Could you check a few things on this model? Use its own coordinates, in mm. A direction names the side the tool comes from. Give positions to 0.01 mm unless a question says otherwise; leave off trailing zeros. Loops run counter-clockwise (first coordinate to the right, second up) from the corner with the lowest first, then second, coordinate; pieces in that order, holes last. Notation, with made-up numbers: (84, 5) - (124, 5) arc R30 cw to (124, 31) - close; hole circle Ø5 at (60, 87.5). An arc over 180 degrees is marked (long way). Answer in a Markdown table with one row per item. Add a question column.
```python
from build123d import *

# Parameters (mm, degrees)
SKETCH1_W           = 70.5
SKETCH1_H           = 70.5
SKETCH1_W_2         = 60.5
SKETCH1_H_2         = 60.5
BOSS_EXTRUDE1_DEPTH = 10
SKETCH2_W           = 67
SKETCH2_H           = 5.4
CUT_EXTRUDE1_DEPTH  = 70
BOSS_EXTRUDE3_DEPTH = 2
SKETCH7_W           = 60.5
SKETCH7_H           = 5
CUT_EXTRUDE3_DEPTH  = 25
FILLET2_R           = 2
SKETCH8_W           = 97.382964501
SKETCH8_H           = 35.083557697
CUT_EXTRUDE4_DEPTH  = 2
SKETCH9_R           = 2.15
CUT_EXTRUDE5_DEPTH  = 5
SKETCH10_R          = 3.5
CUT_EXTRUDE6_DEPTH  = 8
FILLET3_R           = 10
FILLET4_R           = 10
FILLET5_R           = 1


# Some blends are built 0.0001 mm under size
with BuildPart() as part:
    # Sketch1 → Boss-Extrude1 (new body)
    with BuildSketch(Plane(origin=(0, 0, 0), x_dir=(1, 0, 0), z_dir=(0, 1, 0))):
        Rectangle(SKETCH1_W, SKETCH1_H)
        Rectangle(SKETCH1_W_2, SKETCH1_H_2, mode=Mode.SUBTRACT)
    extrude(amount=BOSS_EXTRUDE1_DEPTH)

    # Sketch2 → Cut-Extrude1 (cut)
    with BuildSketch(Plane.XY.offset(35.25)):
        Rectangle(SKETCH2_W, SKETCH2_H)
    extrude(amount=-CUT_EXTRUDE1_DEPTH, mode=Mode.SUBTRACT)

    # Sketch6 → Boss-Extrude3 (add)
    with BuildSketch(Plane.XZ):
        Polygon((41.25, -37.25), (41.25, 37.25), (35.25, 37.25), (35.25, 35.25), (35.25, -35.25), (-35.25, -35.25), (-35.25, 35.25), (-35.25, 37.25), (-41.25, 37.25), (-41.25, -37.25), align=None)
    extrude(amount=-BOSS_EXTRUDE3_DEPTH)

    # Sketch7 → Cut-Extrude3 (cut)
    with BuildSketch(Plane.XZ.offset(-2.7)):
        with Locations((0, 32.75)):
            Rectangle(SKETCH7_W, SKETCH7_H)
    extrude(amount=-CUT_EXTRUDE3_DEPTH, mode=Mode.SUBTRACT)

    # Fillet2
    fillet2_edges = [part.edges().sort_by_distance(p)[0] for p in [
        (35.25, 2, 0),
        (-35.25, 2, 0),
        (0, 2, -35.25),
    ]]
    fillet(fillet2_edges, radius=FILLET2_R - 0.0001)  # a hair under: the kernel refuses the full size

    # Sketch8 → Cut-Extrude4 (cut)
    with BuildSketch(Plane.XY.offset(37.25)):
        with Locations((-5.820498703, 2.430952297)):
            Rectangle(SKETCH8_W, SKETCH8_H)
    extrude(amount=-CUT_EXTRUDE4_DEPTH, mode=Mode.SUBTRACT)

    # Sketch9 → Cut-Extrude5 (cut, symmetric)
    with BuildSketch(Plane.XZ):
        with Locations(Location((-37.375, 25.25, 0), (0, 0, 273.333029494))):
            Circle(SKETCH9_R)
        with Locations(Location((-37.375, -19.75, 0), (0, 0, 273.333029494))):
            Circle(SKETCH9_R)
        with Locations(Location((37.375, -19.75, 0), (0, 0, 266.666970506))):
            Circle(SKETCH9_R)
        with Locations(Location((37.375, 25.25, 0), (0, 0, 266.666970506))):
            Circle(SKETCH9_R)
    extrude(amount=CUT_EXTRUDE5_DEPTH, both=True, mode=Mode.SUBTRACT)

    # Sketch10 → Cut-Extrude6 (cut)
    with BuildSketch(Plane(origin=(0, 10, 0), x_dir=(1, 0, 0), z_dir=(0, 1, 0))):
        with Locations((-37.375, 19.75)):
            Circle(SKETCH10_R)
        with Locations((-37.375, -25.25)):
            Circle(SKETCH10_R)
        with Locations((37.375, -25.25)):
            Circle(SKETCH10_R)
        with Locations((37.375, 19.75)):
            Circle(SKETCH10_R)
    extrude(amount=-CUT_EXTRUDE6_DEPTH, mode=Mode.SUBTRACT)

    # Fillet3
    # the kernel refuses this fillet: 10 mm, written as the material it takes off along each edge
    with BuildSketch(Plane(origin=(-33.5, -24.358969087, 35.25), x_dir=(0, 0, -1), z_dir=(0, 1, 0)), Plane(origin=(33.5, 2.7, 35.25), x_dir=(0, 0, -1), z_dir=(0, -1, 0))) as fillet3_piece_1:
        with BuildLine():
            CenterArc((9.743587635, 10), FILLET3_R, 193.002878163, 76.997121837)
            Line((0, 7.75), (0, 0))
            Line((0, 0), (9.743587635, 0))
        make_face()
    extrude(amount=27.058969087, mode=Mode.SUBTRACT)

    # Fillet4
    # the kernel refuses this fillet: 10 mm, written as the material it takes off along each edge
    with BuildSketch(Plane(origin=(30.25, -18.950635095, 35.25), x_dir=(0, 0, -1), z_dir=(0, 1, 0))) as fillet4_piece_1:
        with BuildLine():
            CenterArc((8.660254038, -10), FILLET4_R, 90, 60)
            Line((0, -5), (-0.173205081, -4.9))
            ThreePointArc((-0.173205081, -4.9), (-0.2, -2.5), (-0.2, 0))
            Line((-0.2, 0), (0, 0.2))
            Line((0, 0.2), (8.660254038, 0.2))
            Line((8.660254038, 0.2), (8.660254038, 0))
        make_face()
    extrude(amount=50.601270189, mode=Mode.SUBTRACT)
    with BuildSketch(Plane(origin=(-30.25, -18.950635095, 35.25), x_dir=(0, 0, -1), z_dir=(0, 1, 0))) as fillet4_piece_2:
        with BuildLine():
            CenterArc((8.660254038, 10), FILLET4_R, 210, 60)
            Line((0, 5), (-0.173205081, 4.9))
            ThreePointArc((-0.173205081, 4.9), (-0.2, 2.5), (-0.2, 0))
            Line((-0.2, 0), (0, -0.2))
            Line((0, -0.2), (8.660254038, -0.2))
            Line((8.660254038, -0.2), (8.660254038, 0))
        make_face()
    extrude(amount=50.601270189, mode=Mode.SUBTRACT)

    # Fillet5
    # the kernel refuses this fillet: 1 mm, written as the material it takes off along each edge
    with BuildSketch(Plane(origin=(30.25, 2.7, 26.589745962), x_dir=(1, 0, 0), z_dir=(0, 0, -1)), Plane(origin=(-30.25, 2.7, -30.25), x_dir=(-1, 0, 0), z_dir=(0, 0, 1))) as fillet5_piece_1:
        with BuildLine():
            CenterArc((FILLET5_R, -FILLET5_R), FILLET5_R, 90, 90)
            Line((0, -FILLET5_R), (0, 0))
            Line((0, 0), (FILLET5_R, 0))
        make_face()
    extrude(amount=56.839745962, mode=Mode.SUBTRACT)
    with BuildSketch(Plane(origin=(40.25, 2.7, 26.589745962), x_dir=(-0.27015512952929444, 0, 0.9628168081151316), z_dir=(0.9628168081151316, 0, 0.27015512952929444))) as fillet5_piece_2:
        with BuildLine():
            CenterArc((10 - FILLET5_R, -FILLET5_R), FILLET5_R, 0, 90)
            Line((10 - FILLET5_R, 0), (10, 0))
            Line((10, 0), (10, -FILLET5_R))
        make_face()
    revolve(axis=Axis((40.25, 2.7, 26.589745962), (0, -1, 0)), revolution_arc=74.326501832, mode=Mode.SUBTRACT)
    with BuildSketch(Plane(origin=(-40.25, 2.7, 26.589745962), x_dir=(1, 0, 0), z_dir=(0, 0, -1))) as fillet5_piece_3:
        with BuildLine():
            CenterArc((10 - FILLET5_R, -FILLET5_R), FILLET5_R, 0, 90)
            Line((10, -FILLET5_R), (10, 0))
            Line((10, 0), (10 - FILLET5_R, 0))
        make_face()
    revolve(axis=Axis((-40.25, 2.7, 26.589745962), (0, -1, 0)), revolution_arc=74.326501832, mode=Mode.SUBTRACT)


solid = part.part
```
(1) I want a section at D-D on y = 5.75. Please give me the cut outline in (x, z) (3 decimals), then the cut area to 3 significant figures.
(2) For pin 1 Ø3 at (y, z) = (7.5, -31) entering from -X; pin 2 Ø6 at (x, y) = (-16, 5) entering from +Z; pin 3 Ø1 at (y, z) = (3, 12) entering from -X; pin 4 Ø3.5 at (x, z) = (-37.375, 25.25) entering from +Y, each with a flat end and sliding along its axis, tell me the tip position at first contact or that it passes through.
(3) Please list where these lines run through material, in increasing order: line 1 (X direction, y = 0.9, z = -19.75) (3 decimals); line 2 (X direction, y = 7, z = -5); line 3 (X direction, y = 1, z = -5).
(4) On a 3-axis mill with a long thin cutter (end or side, diameter ignored), from which of +Z, -Z, +X, -X, +Y, -Y can I reach the whole of each face in a straight line? I mean faces 1 (the cylindrical face through (33.876, 6.056, 25.175)), 2 (the cylindrical face through (-33.876, 6.056, 25.325)), 3 (the flat face through (35.25, 7, 32)), 4 (the flat face through (0, 1, -34.75)). Say none if no direction works.
(5) I want a section at B-B on z = 13. Please give me the cut outline in (x, y).
(6) I want a section at A-A on z = -19.75. Please give me the cut outline in (x, y) (3 decimals).
Reported:
| question | item | result |
|---|---|---|
| 1 | outline | (-35.25, -35.25) - (35.25, -35.25) - (35.25, -22.531) arc R3.5 cw to (35.25, -16.969) - (35.25, 22.469) arc R3.5 cw to (35.25, 28.031) - (35.25, 35.25) arc R10 ccw to (30.25, 26.59) - (30.25, -30.25) - (-30.25, -30.25) - (-30.25, 26.59) arc R10 ccw to (-35.25, 35.25) - (-35.25, 28.031) arc R3.5 cw to (-35.25, 22.469) - (-35.25, -16.969) arc R3.5 cw to (-35.25, -22.531) - close |
| 1 | area | 961 mm² |
| 2 | pin 1 | x = -35.25 |
| 2 | pin 2 | z = -30.25 |
| 2 | pin 3 | x = -35.93 |
| 2 | pin 4 | through |
| 3 | line 1 | -41.25 to -39.525, -35.225 to -33.5, 33.5 to 35.225, 39.525 to 41.25 |
| 3 | line 2 | -35.25 to -30.25, 30.25 to 35.25 |
| 3 | line 3 | -41.25 to -33.5, 33.5 to 41.25 |
| 4 | face 1 | +X, +Y |
| 4 | face 2 | -X, +Y |
| 4 | face 3 | +Z, -Z, +X, +Y |
| 4 | face 4 | +Z, -Y |
| 5 | outline | (-41.25, 0) - (-33.5, 0) - (-33.5, 2.7) - (-31.25, 2.7) arc R1 ccw to (-30.25, 3.7) - (-30.25, 10) - (-35.25, 10) - (-35.25, 4) arc R2 cw to (-37.25, 2) - (-41.25, 2) - close; (30.25, 3.7) arc R1 ccw to (31.25, 2.7) - (33.5, 2.7) - (33.5, 0) - (41.25, 0) - (41.25, 2) - (37.25, 2) arc R2 cw to (35.25, 4) - (35.25, 10) - (30.25, 10) - close |
| 6 | outline | (-41.25, 0) - (-39.525, 0) - (-39.525, 2) - (-41.25, 2) - close; (-35.225, 0) - (-33.5, 0) - (-33.5, 2.7) - (-31.25, 2.7) arc R1 ccw to (-30.25, 3.7) - (-30.25, 10) - (-33.875, 10) - (-33.875, 2) - (-35.225, 2) - close; (30.25, 3.7) arc R1 ccw to (31.25, 2.7) - (33.5, 2.7) - (33.5, 0) - (35.225, 0) - (35.225, 2) - (33.875, 2) - (33.875, 10) - (30.25, 10) - close; (39.525, 0) - (41.25, 0) - (41.25, 2) - (39.525, 2) - close |
